Autodesk Inventor part; units mm, degrees
ref_plane "YZ Plane" through (0, 0, 0) normal (1, 0, 0) x (0, 1, 0)
ref_plane "XZ Plane" through (0, 0, 0) normal (0, 1, 0) x (-1, 0, 0)
ref_plane "XY Plane" through (0, 0, 0) normal (0, 0, 1) x (1, 0, 0)
sketch "Эскиз1" plane through (0, 0, 0) normal (0, 1, 0) x (-1, 0, 0)
  line L0 (0, 0) -> (14.1, 0)
  line L1 (14.1, 0) -> (14.1, -6)
  line L2 (14.1, -6) -> (0, -6)
  line L3 (0, -6) -> (0, 0)
  dimension "d0" = 14.1
  dimension "d1" = 6
extrude "Выдавливание1" add sketch "Эскиз1" along normal blind 10.5
sketch "Эскиз2" plane through (0, 10.5, 0) normal (0, 1, 0) x (1, 0, 0)
  line L0 (-14.1, 0) -> (0, 0)
  line L1 (-7.05, 0) -> (-7.05, 2.075)
  dimension "d4" = 2.075
hole "Отверстие1" at (-7.05, 10.5, -2.075) direction (0, -1, 0) diameter 2 depth 5 tip angle 118
sketch "Эскиз3" plane through (0, 0, 0) normal (0, -1, 0) x (1, 0, 0)
  line L0 (0, 0) -> (0, -6)
  line L1 (0, -3) -> (-3.05, -3)
  line L2 (-14.1, -6) -> (-14.1, 0)
  line L3 (-14.1, -3) -> (-11.05, -3)
  line L4 (0, 0) -> (0, -6)
  line L5 (-14.1, -6) -> (-14.1, 0)
  line L6 (-14.1, 0) -> (0, 0)
  dimension "d12" = 3
  dimension "d24" = 8
hole "Отверстие2" at (-3.05, 0, -3) at (-11.05, 0, -3) direction (0, 1, 0) diameter 2.2 depth 5
sketch "Эскиз4" plane through (0, 0, 0) normal (0, -1, 0) x (1, 0, 0)
  circle A0 centre (-3.05, -3) radius 1.1
  circle A1 centre (-11.05, -3) radius 1.1
  line L0 (-3.05, -5.1939) -> (-4.95, -4.097)
  line L1 (-4.95, -4.097) -> (-4.95, -1.903)
  line L2 (-4.95, -1.903) -> (-3.05, -0.8061)
  line L3 (-3.05, -0.8061) -> (-1.15, -1.903)
  line L4 (-1.15, -1.903) -> (-1.15, -4.097)
  line L5 (-1.15, -4.097) -> (-3.05, -5.1939)
  line L6 (0, 0) -> (0, -6)
  line L7 (-11.05, -5.1939) -> (-12.95, -4.097)
  line L8 (-12.95, -4.097) -> (-12.95, -1.903)
  line L9 (-12.95, -1.903) -> (-11.05, -0.8061)
  line L10 (-11.05, -0.8061) -> (-9.15, -1.903)
  line L11 (-9.15, -1.903) -> (-9.15, -4.097)
  line L12 (-9.15, -4.097) -> (-11.05, -5.1939)
  line L13 (-1.15, -1.903) -> (-4.95, -1.903)
  line L14 (-4.95, -1.903) -> (-4.95, 0)
  line L15 (-4.95, 0) -> (-1.15, 0)
  line L16 (-1.15, 0) -> (-1.15, -1.903)
  line L17 (-14.1, 0) -> (0, 0)
  line L18 (-9.15, -1.903) -> (-12.95, -1.903)
  line L19 (-12.95, -1.903) -> (-12.95, 0)
  line L20 (-12.95, 0) -> (-9.15, 0)
  line L21 (-9.15, 0) -> (-9.15, -1.903)
  point P0 (-3.05, 0)
  point P1 (-9.15, 0)
  dimension "d21" = 3.8
extrude "Выдавливание2" cut sketch "Эскиз4" along normal blind 2 from surface at -5
chamfer "Фаска1" distance 0.8 distance2 6.15 1 edges at (-14.1, 10.5, -3) measured on face at (-7.05, 10.5, -5.025)
chamfer "Фаска2" distance 0.8 distance2 6.15 1 edges at (0, 10.5, -3) measured on face at (-6.7833, 10.5, -5.025)
chamfer "Фаска3" distance 1.5 distance2 6.15 1 edges at (-7.05, 10.5, -6) measured on face at (-7.05, 10.5, -5.025)
equation "\"Радиус_гибки\" = Толщина"
equation "\"Ширина_просечки\" = Толщина"
equation "\"Глубина_просечки\" = 0.5 * Толщина"
equation "\"Размер_просечки\" = 4 * Толщина"
equation "\"Мин_остаток\" = 2 * Толщина"
equation "\"Радиус_перехода\" = Радиус_гибки"
equation "\"Радиус_Якоби\" = Толщина"
equation "\"Размер_зазора\" = Толщина"
properties part number "Съемная стойка сервы"
Work out the finished part from the listing and answer in its coordinate system (mm). A direction names the side the tool comes from. Give positions to 0.01 mm unless a question says otherwise; leave off trailing zeros. Loops run counter-clockwise (first coordinate to the right, second up) from the corner with the lowest first, then second, coordinate; pieces in that order, holes last. Notation, with made-up numbers: (-0.75, 49) -> (55.25, 49) arc R7 cw to (55.25, 54) -> close; hole circle Ø7 at (81, 36). An arc over 180 degrees is marked (long way). One line per question, with ' | ' between items. Start each with the question number.
1) For faces 1 (the face through (-7.35, 7.96, -1.12)), 2 (the face through (-7, 0, -3)), 3 (the face through (-3, 5, -3)), 4 (the face through (-11.98, 1.52, -3.59)), determine the directions among +Z, -Z, +X, -X, +Y, -Y from which every point of the face is accessible in a straight line to the end or side of a thin tool.
2) Determine the mould class of faces 5 (the face through (-0.394, 7.382, -2.375)), 6 (the face through (-2.09, 4.01, -4.64)), 7 (the face through (-7.042, 5.003, -2.248)) for opening direction Z: +Z half, -Z half, draft (parallel to the pull), parting line (faces both ways), or undercut.
3) Section D-D, the plane x = -1.5 is taken. Determine the outline of the cut face in (y, z).
4) Each of these flat-tipped pins is pushed along its axis until it touches: pin 1 (1.8 mm diameter, centred on x = -3.05, z = -3, fed in from -Y); pin 2 (2 mm diameter, centred on y = 8, z = -2.5, fed in from -X). Where does it stop, or does it pass through?
5) Section C-C, the plane x = -11.5 is taken. Determine the outline of the cut face in (y, z).
6) Straight lines are drawn through the part: L1, parallel to X at y = 2.4, z = -3; L2, parallel to Y at x = -4.75, z = -3.5; L3, parallel to Z at x = -11.05, y = 1.15. For each, find the intervals that lie inside material, in ascending order.
7) Section B-B, the plane y = 1.75 is taken. Determine the outline of the cut face in (x, z).
8) Section A-A, the plane y = 4 is taken. Determine the outline of the cut face in (x, z).
Resolved:
1) face 1: +Y | face 2: +Z, -Z, +X, -X, -Y | face 3: +Z | face 4: -Y
2) face 5: draft | face 6: +Z half | face 7: undercut
3) outline: (0, -6) -> (4.35, -6) -> (10.5, -4.5) -> (10.5, 0) -> (5, 0) -> (5, -4.3) -> (3, -4.3) -> (3, 0) -> (0, 0) -> close
4) pin 1: y = 5 | pin 2: x = -13.76
5) outline: (0, -6) -> (4.35, -6) -> (10.5, -4.5) -> (10.5, 0) -> (5, 0) -> (5, -4.93) -> (3, -4.93) -> (3, -4) -> (0, -4) -> close; (0, -2) -> (3, -2) -> (3, 0) -> (0, 0) -> close
6) L1: -14.1 to -12.15, -9.95 to -4.15, -1.95 to 0 | L2: 0 to 3, 5 to 10.5 | L3: -6 to -4.1, -1.9 to 0
7) outline: (-14.1, -6) -> (0, -6) -> (0, 0) -> (-14.1, 0) -> close; hole circle Ø2.2 at (-11.05, -3); hole circle Ø2.2 at (-3.05, -3)
8) outline: (-14.1, -6) -> (0, -6) -> (0, 0) -> (-1.15, 0) -> (-1.15, -4.1) -> (-3.05, -5.19) -> (-4.95, -4.1) -> (-4.95, 0) -> (-9.15, 0) -> (-9.15, -4.1) -> (-11.05, -5.19) -> (-12.95, -4.1) -> (-12.95, 0) -> (-14.1, 0) -> close
